Verification items for the finished model (mm, model axes). A direction names the side the tool comes from. Round coordinates to 2 decimals unless told otherwise and drop trailing zeros. Write each loop counter-clockwise with the first axis right and the second up, starting at its lowest first coordinate (ties: lowest second). Pieces come first, ordered by that corner, then holes. Notation, with made-up numbers: M 69,-13 L 80,-13 A9 ccw 80,4 Z; hole C 88.25,22 d1. An arc over 180 degrees is marked long. Answer in a Markdown table with one row per item. Add a question column.
1. Go/stop test with flat-tipped pins: pin 1 Ø3 at (x, y) = (4.5, 1) entering from -Z; pin 2 Ø0.8 at (x, y) = (0.5, 0) entering from -Z; pin 3 Ø4 at (x, y) = (7, -1.5) entering from +Z. Record where each tip stops, or that it passes through.
2. Set-up check for faces 4 (the flat face through (0.49, -0.87, 0.49)), 5 (the flat face through (0, 1, -1)), 6 (the cylindrical face through (5.242, -1.617, 0.67)): record each of +Z, -Z, +X, -X, +Y, -Y from which the full face is reachable in a straight line by a thin tool's end or side.
3. Draft check along X on faces 1 (the flat face through (0.49, 0.87, -0.49)), 2 (the flat face through (8.2, 0, 0)), 3 (the flat face through (1, 0, 0)). Enter one of: pulls with the +X half, pulls with the -X half, needs draft (parallel to the pull), parting line crosses it, or undercut.
4. Material ranges on probe 1 along X at (y, z) = (0.75, -2); probe 2 along Z at (x, y) = (6.5, -1); probe 3 along X at (y, z) = (0.25, -2.5), recorded low to high.
5. Sectioned sample at A-A on x = 5.75. Record the cut outline in (y, z).
```python
from build123d import *

# Parameters (mm, degrees)
CUT_EXTRUDE_1_DEPTH = 1


with BuildPart() as part:
    # 草图1 → 旋转1 (revolve)
    with BuildSketch(Plane.XY, mode=Mode.PRIVATE) as revolve_1_sk:
        with BuildLine():
            Line((0, 0), (0, 2.2))
            ThreePointArc((0, 2.2), (0.920270994, 3.188453389), (2.2, 3.62))
            Line((2.2, 3.62), (2.2, 1.75))
            Line((2.2, 1.75), (8.2, 1.75))
            Line((8.2, 1.75), (8.2, 0))
            Line((8.2, 0), (0, 0))
        make_face()
    revolve(revolve_1_sk.sketch.rotate(Axis((0, 0, 0), (1, 0, 0)), 180), axis=Axis((0, 0, 0), (1, 0, 0)))

    # 草图2 → 切除-拉伸1 (cut)
    with BuildSketch(Plane.ZY):
        Polygon((0, 1.154700538), (-1, 0.577350269), (-1, -0.577350269), (0, -1.154700538), (1, -0.577350269), (1, 0.577350269), align=None)
    extrude(amount=-CUT_EXTRUDE_1_DEPTH, mode=Mode.SUBTRACT)


solid = part.part
```
Geometry check:
| question | item | result |
|---|---|---|
| 1 | pin 1 | stops at z = -1.75 |
| 1 | pin 2 | stops at z = -3.18 |
| 1 | pin 3 | stops at z = 1.75 |
| 2 | face 4 | -X |
| 2 | face 5 | +Z, -Z, -X, +Y, -Y |
| 2 | face 6 | +X |
| 3 | face 1 | needs draft |
| 3 | face 2 | pulls with the +X half |
| 3 | face 3 | pulls with the -X half |
| 4 | probe 1 | x = 0 to 2.2 |
| 4 | probe 2 | z = -1.44 to 1.44 |
| 4 | probe 3 | x = 0.2 to 2.2 |
| 5 | outline | C 0,0 d3.5 |
